```python
from build123d import *

# Parameters (mm, degrees)
SKETCH3_R          = 1.75
CUT_EXTRUDE2_DEPTH = 3


with BuildPart() as part:
    # Sketch1 → Revolve1 (revolve)
    with BuildSketch(Plane.XY):
        Polygon((-5.75, -5.1), (-5.75, -11), (-2.75, -11), (-2.75, -5.1), (7.25, -5.1), (7.25, -4), (-7.25, -4), (-7.25, -5.1), align=None)
    revolve(axis=Axis((-7.25, 0, 0), (1, 0, 0)))

    # Sketch3 → Cut-Extrude2 (cut)
    with BuildSketch(Plane.ZY.offset(5.75)):
        with Locations((0, 8)):
            Circle(SKETCH3_R)
        with Locations((0, -8)):
            Circle(SKETCH3_R)
        with Locations((8, 0)):
            Circle(SKETCH3_R)
        with Locations((-8, 0)):
            Circle(SKETCH3_R)
        Polygon((5205.178442712, 2346.745629148), (5205.178442712, 2340.845629148), (5208.178442712, 2340.845629148), (5208.178442712, 2346.745629148), (5218.178442712, 2346.745629148), (5218.178442712, 2347.845629148), (5203.678442712, 2347.845629148), (5203.678442712, 2346.745629148), align=None)
    extrude(amount=-CUT_EXTRUDE2_DEPTH, mode=Mode.SUBTRACT)


solid = part.part
```
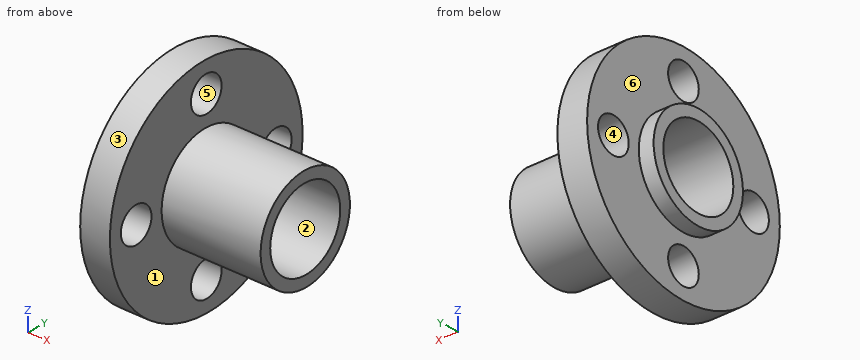
Could you check a few things on this model? Use its own coordinates, in mm. Face numbers are marked on the shaded views. A direction names the side the tool comes from. Round coordinates to 2 decimals unless told otherwise and drop trailing zeros. Loops run counter-clockwise (first coordinate to the right, second up) from the corner with the lowest first, then second, coordinate; pieces in that order, holes last. Notation, with made-up numbers: (68, 40.25) -> (119, 40.25) arc R27 cw to (119, 69.25) -> close; hole circle Ø6 at (85, 87.25). An arc over 180 degrees is marked (long way). One line per question, with ' | ' between items.
(1) For pin 1 Ø7 at (y, z) = (0, 0) entering from -X; pin 2 Ø5.5 at (y, z) = (0, 8) entering from -X; pin 3 Ø4 at (y, z) = (-8, 0) entering from +X; pin 4 Ø1 at (x, y) = (1, 5) entering from +Z, each with a flat end and sliding along its axis, tell me the tip position at first contact or that it passes through.
Model answer:
pin 1: passes through | pin 2: stops at x = -5.75 | pin 3: stops at x = -2.75 | pin 4: stops at z = 2.4
(2) If we section it at D-D on y = 8: List the corners of the cut face in (x, z) for me, and give its area (3 significant figures).
Model answer:
outline: (-5.75, -7.55) -> (-2.75, -7.55) -> (-2.75, -1.75) -> (-5.75, -1.75) -> close; (-5.75, 1.75) -> (-2.75, 1.75) -> (-2.75, 7.55) -> (-5.75, 7.55) -> close | area: 34.8 mm^2
(3) For the marked faces 1 and 2, which set-ups out of +Z, -Z, +X, -X, +Y, -Y let a thin tool reach every point of the face, with its end or its side?
Model answer:
face 1: +X | face 2: +X, -X
(4) If I drill on probe 1 along Z at (x, y) = (-0.5, 0); probe 2 along Y at (x, z) = (-3.4, 0), over which ranges is the centre line in solid material (lowest first)?
Model answer:
probe 1: z = -5.1 to -4, 4 to 5.1 | probe 2: y = -11 to -9.75, -6.25 to -4, 4 to 6.25, 9.75 to 11
(5) If we section it at C-C on x = -3.5: List the corners of the cut face in (y, z) for me.
Model answer:
outline: circle Ø22 at (0, 0); hole circle Ø3.5 at (-8, 0); hole circle Ø8 at (0, 0); hole circle Ø3.5 at (0, -8); hole circle Ø3.5 at (0, 8); hole circle Ø3.5 at (8, 0)
(6) Thinking about a two-plate mould opening in Y: for the marked faces 3, 4, 5 and 6, which applies, released by +Y, released by -Y, zero draft, split by the parting line, or undercut?
Model answer:
face 3: split by the parting line | face 4: undercut | face 5: undercut | face 6: zero draft
(7) If we section it at A-A on z = 0: List the corners of the cut face in (x, y) for me.
Model answer:
outline: (-7.25, -5.1) -> (-5.75, -5.1) -> (-5.75, -6.25) -> (-2.75, -6.25) -> (-2.75, -5.1) -> (7.25, -5.1) -> (7.25, -4) -> (-7.25, -4) -> close; (-7.25, 4) -> (7.25, 4) -> (7.25, 5.1) -> (-2.75, 5.1) -> (-2.75, 6.25) -> (-5.75, 6.25) -> (-5.75, 5.1) -> (-7.25, 5.1) -> close; (-5.75, -11) -> (-2.75, -11) -> (-2.75, -9.75) -> (-5.75, -9.75) -> close; (-5.75, 9.75) -> (-2.75, 9.75) -> (-2.75, 11) -> (-5.75, 11) -> close
